Can you work these out from the drawing? Everything is in mm from the part's minimum corner. Round coordinates to 2 decimals unless told otherwise and drop trailing zeros. Write each loop counter-clockwise with the first axis right and the second up, starting at its lowest first coordinate (ties: lowest second). Pieces come first, ordered by that corner, then holes. Notation, with made-up numbers: (50, 22.25) - (104, 22.25) arc R12 cw to (104, 27.25) - close; hole circle Ø1 at (25.5, -36). An arc over 180 degrees is marked (long way). Write each question's results on one line, items separated by ' | '. Start each with the question number.
(1) Thinking about a two-plate mould opening in Z: for the marked faces 1, 2, 3 and 4, which applies, +Z half, -Z half, draft (parallel to the pull), parting line (faces both ways), or undercut?
(2) Imagine slicing it at A-A on x = 57.15. Write out the boundary of the cut face in (y, z).
(3) Imagine slicing it at B-B on y = 5. State how many separate pieces and enclosed holes the cut face has, then the cut area to 3 significant figures.
(4) Please list where these lines run through material, in increasing order: line 1 (X direction, y = 1, z = 17.25) (1 decimal); line 2 (Z direction, x = 57.15, y = 2.25); line 3 (X direction, y = 5, z = 14.25). Write a range as [from, to].
(5) For P1, Ø11, axis at x = 19.05, z = 15.875, coming from the +Y side, with a flat end and sliding along its axis, tell me the tip position at first contact or that it passes through.
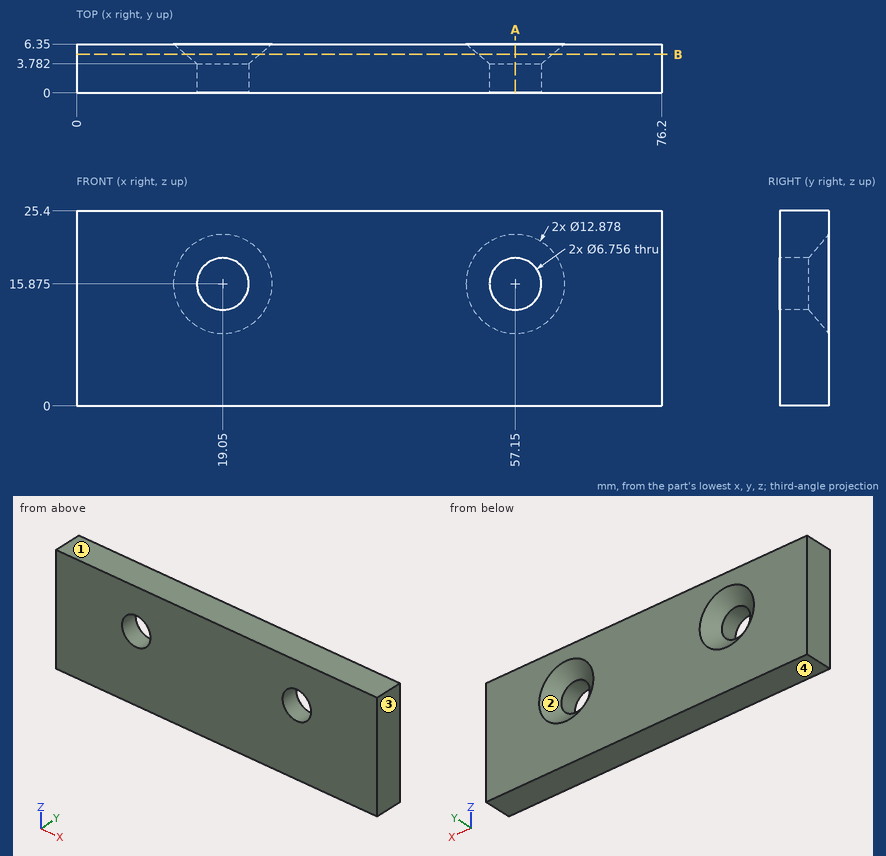
Response:
1) face 1: +Z half | face 2: undercut | face 3: draft | face 4: -Z half
2) outline: (0, 0) - (6.35, 0) - (6.35, 9.44) - (3.78, 12.5) - (0, 12.5) - close; (0, 19.25) - (3.78, 19.25) - (6.35, 22.31) - (6.35, 25.4) - (0, 25.4) - close
3) separate pieces: 1 | enclosed holes: 2 | area: 1,790 mm²
4) line 1: [0, 16], [22.1, 54.1], [60.2, 76.2] | line 2: [0, 12.5], [19.25, 25.4] | line 3: [0, 14.5], [23.6, 52.6], [61.7, 76.2]
5) P1: y = 5.56
